from build123d import *

# Parameters (mm, degrees)
F2_DEPTH = 50
F3_DEPTH = 50


with BuildPart() as f2:
    # F0 (on Top) → F2 (new body, symmetric)
    with BuildSketch(Plane.XY):
        Polygon((-20, 50), (-50, 50), (-15, 0), (-15, -50), (15, -50), (15, 0), (50, 50), (20, 50), (0, 20), align=None)
    extrude(amount=F2_DEPTH, both=True)

    # F1 (on Front) → F3 (intersect, symmetric)
    with BuildSketch(Plane.XZ):
        with BuildLine():
            ThreePointArc((-40.222977, 50.086129), (-47.329808, 47.143242), (-50.244602, 40.024844))
            Line((-50.244602, 40.024844), (-49.754141, -39.972961))
            ThreePointArc((-49.754141, -39.972961), (-46.811419, -46.996671), (-39.776142, -49.911629))
            Line((-39.776142, -49.911629), (-29.693388, -49.933623))
            ThreePointArc((-29.693388, -49.933623), (-22.615948, -47.020121), (-19.671599, -39.955459))
            Line((-19.671599, -39.955459), (-19.649794, -29.958878))
            ThreePointArc((-19.649794, -29.958878), (-16.705445, -22.894216), (-9.628005, -19.980714))
            Line((-9.628005, -19.980714), (49.638809, -20.109991))
            Line((49.638809, -20.109991), (49.638809, 4.890009))
            Line((49.638809, 4.890009), (-9.67163, 5.019381))
            ThreePointArc((-9.67163, 5.019381), (-16.736293, 7.96373), (-19.649794, 15.04117))
            ThreePointArc((-19.649794, 15.04117), (-16.705445, 22.105832), (-9.628005, 25.019333))
            Line((-9.628005, 25.019333), (49.638809, 24.890057))
            Line((49.638809, 24.890057), (49.69334, 49.889997))
            Line((49.69334, 49.889997), (-40.222977, 50.086129))
        make_face()
    extrude(amount=F3_DEPTH, both=True, mode=Mode.INTERSECT)


solid = f2.part
For this review, take the finished solid that the model builds, in its own axes (mm). A direction names the side the tool comes from. Give positions to 0.01 mm unless a question says otherwise; leave off trailing zeros. Order: outer loops, then holes, each group sorted by start corner. A loop starts at its lowest first (then second) coordinate and runs counter-clockwise, first axis right, second up. Notation, with made-up numbers: M -7,10 L 24,10 A23 ccw 24,35 Z; hole C -12.75,-1 d1. An arc over 180 degrees is marked long. Answer in a Markdown table with one row per item. Add a question column.
(1) Wall thickness on probe 1 along Z at (x, y) = (10.5, -41); probe 2 along Y at (x, z) = (-29, -27); probe 3 along X at (y, z) = (-20.5, -4): over which ranges is each line inside the solid? List them lowest first. Write a range as [from, to].
(2) For pin 1 (1 mm diameter, centred on x = 18.5, z = -6.5, fed in from +Y); pin 2 (12 mm diameter, centred on y = -31, z = 8.5, fed in from +X); pin 3 (8.5 mm diameter, centred on y = -37.5, z = -13.5, fed in from -X); pin 4 (8 mm diameter, centred on x = -2.5, y = 38, fed in from +Z), all flat-tipped, find the tip position at first contact; note any pin that passes through.
(3) Consider section C-C on z = -37.5. State the section outline as (x, y) points.
(4) Consider section B-B on x = 13.5. State the section outline as (y, z) points, and give its area (3 significant figures).
(5) Consider section A-A on y = -36.5. State the section outline as (x, z) points, and give its area (3 significant figures).
(6) Consider section D-D on x = 39. State the section outline as (y, z) points.
(7) For faces 1 (the face through (-17, 12, 50)), 2 (the face through (10, 35, 38)), 3 (the face through (-15, -25, 37)), 4 (the face through (15, -25, -7)), list the 3-axis set-ups (+Z, -Z, +X, -X, +Y, -Y) from which the entire face can be reached by the end or side of a thin tool; tool diameter is ignored.
Evaluation:
| question | item | result |
|---|---|---|
| 1 | probe 1 | z = [-20.02, 4.98], [24.98, 49.98] |
| 1 | probe 2 | y = [20, 50] |
| 1 | probe 3 | x = [-15, 15] |
| 2 | pin 1 | stops at y = 48.5 |
| 2 | pin 2 | stops at x = 15 |
| 2 | pin 3 | stops at x = -15 |
| 2 | pin 4 | passes through |
| 3 | outline | M -49.77,49.67 L -19.67,6.67 L -19.67,49.5 L -20,50 L -49.77,50 Z |
| 4 | outline | M -50,-20.03 L 40.25,-20.03 L 40.25,4.97 L -50,4.97 Z; M -50,24.97 L 40.25,24.97 L 40.25,49.97 L -50,49.97 Z |
| 4 | area | 4,510 mm^2 |
| 5 | outline | M -15,-21.53 A10 cw -9.63,-19.98 L 15,-20.03 L 15,4.97 L -9.67,5.02 A10 cw -15,6.57 Z; M -15,23.47 A10 cw -9.63,25.02 L 15,24.97 L 15,49.97 L -0.74,50 L -15,50 Z |
| 5 | area | 1,510 mm^2 |
| 6 | outline | M 34.29,-20.09 L 50,-20.09 L 50,4.91 L 34.29,4.91 Z; M 34.29,24.91 L 50,24.91 L 50,49.91 L 34.29,49.91 Z |
| 7 | face 1 | +Z, +X, -X, +Y, -Y |
| 7 | face 2 | +Z, -Z, +Y |
| 7 | face 3 | +Z, -Z, -X, -Y |
| 7 | face 4 | +Z, -Z, +X, -Y |
